Here's how the part is built. I have some questions about the finished solid (model axes, mm). Face numbers are marked on the shaded views. Round coordinates to 2 decimals unless told otherwise and drop trailing zeros. Write each loop counter-clockwise with the first axis right and the second up, starting at its lowest first coordinate (ties: lowest second). Pieces come first, ordered by that corner, then holes. Notation, with made-up numbers: (-37, 70.5) -> (4, 70.5) arc R21 cw to (4, 79.5) -> close; hole circle Ø2 at (-24, 76). An arc over 180 degrees is marked (long way). Answer in a Markdown table with one row per item.
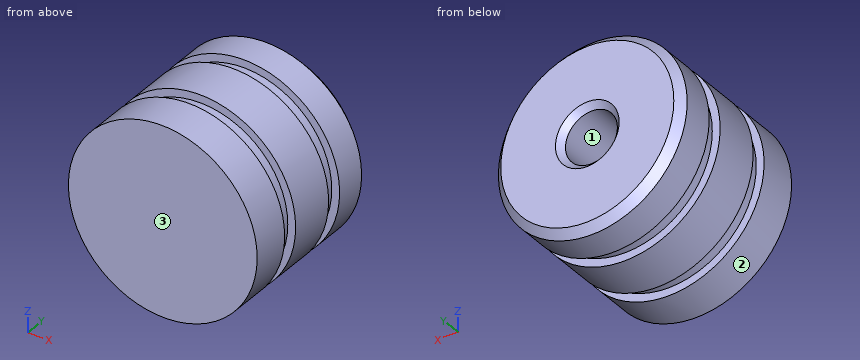
from build123d import *

# Parameters (mm, degrees)
SKETCH1_R                       = 6
BOSS_EXTRUDE1_DEPTH             = 5
CUT_EXTRUDE1_START              = -2.5
SKETCH2_R                       = 6
SKETCH2_R_2                     = 5.5
CUT_EXTRUDE1_DEPTH              = 1
CHAMFER1_SIZE                   = 0.5
M4X0_7_TAPPED_HOLE1_D           = 3.3
M4X0_7_TAPPED_HOLE1_DEPTH       = 8
M4X0_7_TAPPED_HOLE1_CSINK_D     = 4.05
M4X0_7_TAPPED_HOLE1_CSINK_ANGLE = 90
M4X0_7_TAPPED_HOLE1_TIP         = 0.991420021


with BuildPart() as part:
    # Sketch1 → Boss-Extrude1 (new body, symmetric)
    with BuildSketch(Plane(origin=(0, 0, 0), x_dir=(1, 0, 0), z_dir=(0, 1, 0))):
        Circle(SKETCH1_R)
    extrude(amount=BOSS_EXTRUDE1_DEPTH, both=True)

    # Sketch2 → Cut-Extrude1 (cut)
    with BuildSketch(Plane(origin=(0, 5, 0), x_dir=(1, 0, 0), z_dir=(0, 1, 0)).offset(CUT_EXTRUDE1_START)):
        Circle(SKETCH2_R)
        Circle(SKETCH2_R_2, mode=Mode.SUBTRACT)
    cut_extrude1 = extrude(amount=-CUT_EXTRUDE1_DEPTH, mode=Mode.SUBTRACT)

    # Mirror1: Cut-Extrude1 across plane
    add(cut_extrude1.mirror(Plane.ZX), mode=Mode.SUBTRACT)

    # Chamfer1
    chamfer1_edges = [part.edges().sort_by_distance(p)[0] for p in [
        (-6, 5, 0),
    ]]
    chamfer(chamfer1_edges, length=CHAMFER1_SIZE)

    # M4x0.7 Tapped Hole1
    with Locations(Plane(origin=(0, 5, 0), x_dir=(1, 0, 0), z_dir=(0, 1, 0))):
        with Locations((0, 0)):
            CounterSinkHole(M4X0_7_TAPPED_HOLE1_D / 2, M4X0_7_TAPPED_HOLE1_CSINK_D / 2, depth=M4X0_7_TAPPED_HOLE1_DEPTH, counter_sink_angle=M4X0_7_TAPPED_HOLE1_CSINK_ANGLE)
            with Locations((0, 0, -(M4X0_7_TAPPED_HOLE1_DEPTH + M4X0_7_TAPPED_HOLE1_TIP / 2))):  # 118° drill point
                Cone(0, M4X0_7_TAPPED_HOLE1_D / 2, M4X0_7_TAPPED_HOLE1_TIP, mode=Mode.SUBTRACT)


solid = part.part
1) We'd pull the mould along Z, two halves only. Please class the marked faces 1, 2 and 3: +Z half, -Z half, draft (parallel to the pull), parting line (faces both ways), or undercut.
Response:
| item | result |
|---|---|
| face 1 | undercut |
| face 2 | parting line |
| face 3 | draft |
2) For pin 1 (3 mm diameter, centred on x = -4.5, y = -2, fed in from -Z); pin 2 (3 mm diameter, centred on x = -4, y = -0.5, fed in from -Z); pin 3 (2 mm diameter, centred on y = 2.5, z = -3.5, fed in from +X), each with a flat end and sliding along its axis, tell me the tip position at first contact or that it passes through.
Response:
| item | result |
|---|---|
| pin 1 | stops at z = -5.15 |
| pin 2 | stops at z = -5.45 |
| pin 3 | stops at x = 5.45 |
3) I want a section at A-A, the plane y = 0. List the corners of the cut face in (x, z) for me, and give its area (3 significant figures).
Response:
| item | result |
|---|---|
| outline | circle Ø12 at (0, 0); hole circle Ø3.3 at (0, 0) |
| area | 105 mm^2 |
4) I want a section at B-B, the plane y = 2.25. List the corners of the cut face in (x, z) for me.
Response:
| item | result |
|---|---|
| outline | circle Ø11 at (0, 0); hole circle Ø3.3 at (0, 0) |
5) I need wall thicknesses on line 1 (Y direction, x = -5.5, z = -2); line 2 (Z direction, x = 0, y = -1); line 3 (Z direction, x = 0.5, y = 2.25). Which ranges of each line are inside material? Lowest first, please. Write a range as [from, to].
Response:
| item | result |
|---|---|
| line 1 | y = [-5, -2.5], [-1.5, 1.5], [2.5, 4.65] |
| line 2 | z = [-6, -1.65], [1.65, 6] |
| line 3 | z = [-5.48, -1.57], [1.57, 5.48] |
